```python
from build123d import *

# Parameters (mm, degrees)
BASE_FLANGE1_DEPTH = 10
FILLET1_R          = 3
SKETCH8_R          = 1.5
CUT_EXTRUDE1_DEPTH = 18.549928775
SKETCH9_R          = 1
CUT_EXTRUDE2_DEPTH = 18.549928775


# Sheet-metal steps are written as plain solids
with BuildPart() as part:
    # Sketch2 → Base-Flange1 (new, symmetric)
    with BuildSketch(Plane.XY):
        with BuildLine():
            Line((-12, 0), (-0.75, 0))
            ThreePointArc((-0.75, 0), (-0.219669914, 0.219669914), (0, 0.75))
            Line((0, 0.75), (0, 8))
            Line((0, 8), (2, 8))
            Line((2, 8), (2, 0.75))
            ThreePointArc((2, 0.75), (1.194543648, -1.194543648), (-0.75, -2))
            Line((-0.75, -2), (-12, -2))
            Line((-12, -2), (-12, 0))
        make_face()
    extrude(amount=BASE_FLANGE1_DEPTH, both=True)

    # Fillet1
    fillet1_edges = [part.edges().sort_by_distance(p)[0] for p in [
        (-12, -1, 10),
        (1, 8, 10),
        (-12, -1, -10),
        (1, 8, -10),
    ]]
    fillet(fillet1_edges, radius=FILLET1_R)

    # Sketch8 → Cut-Extrude1 (cut, through all)
    with BuildSketch(Plane(origin=(0, 0, 0), x_dir=(1, 0, 0), z_dir=(0, 1, 0))):
        with Locations(Location((-9, 6, 0), (0, 0, 270))):
            Circle(SKETCH8_R)
        with Locations(Location((-9, -6, 0), (0, 0, 90))):
            Circle(SKETCH8_R)
    extrude(amount=-CUT_EXTRUDE1_DEPTH, mode=Mode.SUBTRACT)

    # Sketch9 → Cut-Extrude2 (cut, through all)
    with BuildSketch(Plane.ZY):
        with Locations((0, 6)):
            Circle(SKETCH9_R)
    extrude(amount=-CUT_EXTRUDE2_DEPTH, mode=Mode.SUBTRACT)


solid = part.part
```
CAD build for the part. Positions are in the model's coordinates, mm. A direction names the side the tool comes from. Round coordinates to 2 decimals unless told otherwise and drop trailing zeros. Loops run counter-clockwise (first coordinate to the right, second up) from the corner with the lowest first, then second, coordinate; pieces in that order, holes last. Notation, with made-up numbers: M -33.5,82 L 25.5,82 A10 ccw 25.5,86 Z; hole C -15,33.25 d9. An arc over 180 degrees is marked long. Return JSON: item names as keys, results as strings. Group by question number.
(1) Mould opens along Z. For faces 3 (the cylindrical face through (-11.1, -0.99, 9.14)), 4 (the cylindrical face through (1.22, -1.17, 0.14)), 5 (the cylindrical face through (-7.536, -0.986, 6.325)) say: +Z half, -Z half, draft (parallel to the pull), parting line (faces both ways), or undercut.
(2) Saw through at D-D, the plane z = 4.25. List the corners of the cut face in (x, y).
(3) Drop flat-ended pins along their axis: P1, Ø1, axis at x = -2.5, z = -2, coming from the +Y side; P2, Ø1, axis at x = -3, y = 1, coming from the +Z side; P3, Ø2.5, axis at y = 6, z = 0, coming from the +X side. Give the stop position or say it passes through.
(4) Saw through at A-A, the plane z = 0. List the corners of the cut face in (x, y), and give its area (3 significant figures).
(5) Wall check: probe 1 along Y at (x, z) = (-4.75, 4.5); probe 2 along Z at (x, y) = (-8.75, -1.25); probe 3 along Y at (x, z) = (1.25, -0.75). Give the ranges that are in metal, low to high. Write a range as [from, to].
(6) Tool access for faces 1 (the flat face through (1, 8, 0)), 2 (the flat face through (-6, 0, 0)): list every direction of +Z, -Z, +X, -X, +Y, -Y with a clear straight run to the whole face (end or side of a thin tool).
(7) Saw through at C-C, the plane y = 6. List the corners of the cut face in (x, z), and give its area (3 significant figures).
(8) Saw through at B-B, the plane x = -8.75. List the corners of the cut face in (y, z), and give its area (3 significant figures).
Answer list:
{
 "1": {"face 3": "+Z half", "face 4": "draft", "face 5": "undercut"},
 "2": {"outline": "M -12,-2 L -0.75,-2 A2.75 ccw 2,0.75 L 2,8 L 0,8 L 0,0.75 A0.75 cw -0.75,0 L -12,0 Z"},
 "3": {"P1": "y = 0", "P2": "through", "P3": "x = 2"},
 "4": {"outline": "M -12,-2 L -0.75,-2 A2.75 ccw 2,0.75 L 2,5 L 0,5 L 0,0.75 A0.75 cw -0.75,0 L -12,0 Z; M 0,7 L 2,7 L 2,8 L 0,8 Z", "area": "38.5 mm2"},
 "5": {"probe 1": "[-2, 0]", "probe 2": "[-10, -7.48], [-4.52, 4.52], [7.48, 10]", "probe 3": "[-1.14, 5.34], [6.66, 8]"},
 "6": {"face 1": "+Z, -Z, +X, -X, +Y", "face 2": "+Z, -Z, -X, +Y"},
 "7": {"outline": "M 0,-9.83 L 2,-9.83 L 2,-1 L 0,-1 Z; M 0,1 L 2,1 L 2,9.83 L 0,9.83 Z", "area": "35.3 mm2"},
 "8": {"outline": "M -2,-10 L 0,-10 L 0,-7.48 L -2,-7.48 Z; M -2,-4.52 L 0,-4.52 L 0,4.52 L -2,4.52 Z; M -2,7.48 L 0,7.48 L 0,10 L -2,10 Z", "area": "28.2 mm2"}
}
